from build123d import *

# Parameters (mm, degrees)
BOSS_EXTRUDE1_DEPTH = 20
SKETCH3_W           = 47.8415773
SKETCH3_H           = 21.769183321
SKETCH3_W_2         = 54.74945498
SKETCH3_H_2         = 26.072393978
BOSS_EXTRUDE2_DEPTH = 20


with BuildPart() as part:
    # Sketch1 → Boss-Extrude1 (new body)
    with BuildSketch(Plane.XY):
        Polygon((-57.85830676, 0), (-57.85830676, 45.936170213), (35.982726675, 45.936170213), (35.982726675, -85.966261398), (16.952027587, -85.966261398), (16.952027587, 0), (-37.187030164, 0), (-37.187030164, -22.639969605), (-57.85830676, -22.639969605), align=None)
    extrude(amount=BOSS_EXTRUDE1_DEPTH)

    # Sketch3 → Boss-Extrude2 (add)
    with BuildSketch(Plane.XY):
        with Locations((-45.869735372, -22.040085901)):
            Rectangle(SKETCH3_W, SKETCH3_H)
        with Locations((27.37472749, -83.170990229)):
            Rectangle(SKETCH3_W_2, SKETCH3_H_2)
    extrude(amount=BOSS_EXTRUDE2_DEPTH)


solid = part.part
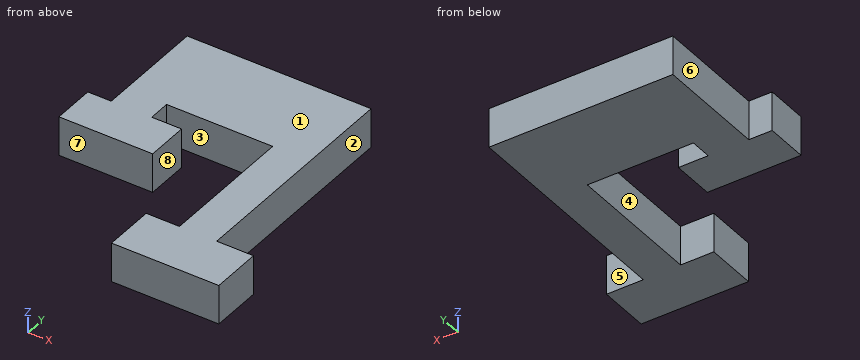
The model under review builds one solid part; all positions refer to its coordinate system, in mm. Face numbers are marked on the shaded views. A direction names the side the tool comes from. Give positions to 0.01 mm unless a question says otherwise; leave off trailing zeros. Write each loop counter-clockwise with the first axis right and the second up, starting at its lowest first coordinate (ties: lowest second). Pieces come first, ordered by that corner, then holes.
1. Tool access review of the marked faces 4, 5, 6, 7 and 8: name each direction out of +Z, -Z, +X, -X, +Y, -Y from which nothing blocks a thin tool from reaching the whole face with its end or side.
2. Add section C-C, the plane z = 17.5. Write out the cut boundary in (x, y), plus the area to 3 significant figures.
3. Add section A-A, the plane x = 12.5. Write out the cut boundary in (y, z).
4. Wall thickness on L1, parallel to Y at x = 14, z = 14; L2, parallel to X at y = -17.5, z = 13.5; L3, parallel to Y at x = -26, z = 11: over which ranges is each line inside the solid? List them lowest first.
5. Add section D-D, the plane x = -13.5. Write out the cut boundary in (y, z), plus the area to 3 significant figures.
6. Draft analysis for pull direction X (two halves, no side actions). For the marked faces 1, 2 and 3, state which applies: +X half, -X half, draft (parallel to the pull), parting line (faces both ways), or undercut.
7. Add section B-B, the plane y = -2.5. Write out the cut boundary in (x, z), plus the area to 3 significant figures.
8. For P1, Ø4, axis at y = 31.5, z = 11, coming from the +X side; P2, Ø1.5, axis at x = -12.5, z = 15.5, coming from the -Y side; P3, Ø10, axis at x = -42.5, z = 12, coming from the -Y side, all flat-tipped, find the tip position at first contact; note any pin that passes through.
Worked answers:
1. face 4: +Z, -Z
1. face 5: +Z, -Z, +X, +Y
1. face 6: +Z, -Z, -X, +Y
1. face 7: +Z, -Z, -X, -Y
1. face 8: +Z, -Z, -Y
2. outline: (-69.79, -32.92) - (-21.95, -32.92) - (-21.95, -11.16) - (-37.19, -11.16) - (-37.19, 0) - (16.95, 0) - (16.95, -70.13) - (0, -70.13) - (0, -96.21) - (54.75, -96.21) - (54.75, -70.13) - (35.98, -70.13) - (35.98, 45.94) - (-57.86, 45.94) - (-57.86, -11.16) - (-69.79, -11.16) - close
2. area: 8,340 mm2
3. outline: (-96.21, 0) - (-70.13, 0) - (-70.13, 20) - (-96.21, 20) - close; (0, 0) - (45.94, 0) - (45.94, 20) - (0, 20) - close
4. L1: y = -96.21 to -70.13, 0 to 45.94
4. L2: x = -69.79 to -21.95, 16.95 to 35.98
4. L3: y = -32.92 to -11.16, 0 to 45.94
5. outline: (0, 0) - (45.94, 0) - (45.94, 20) - (0, 20) - close
5. area: 919 mm2
6. face 1: draft
6. face 2: +X half
6. face 3: undercut
7. outline: (-57.86, 0) - (-37.19, 0) - (-37.19, 20) - (-57.86, 20) - close; (16.95, 0) - (35.98, 0) - (35.98, 20) - (16.95, 20) - close
7. area: 794 mm2
8. P1: stops at x = 35.98
8. P2: stops at y = 0
8. P3: stops at y = -32.92
